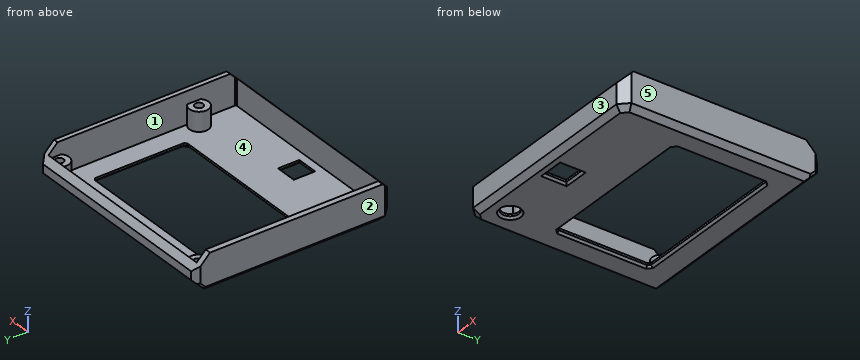
from build123d import *

# Parameters (mm, degrees)
PAD_DEPTH       = 17
POCKET_DEPTH    = 15
SKETCH002_R     = 4
SKETCH002_W     = 74.5
SKETCH002_H     = 43.5
SKETCH002_W_2   = 10
SKETCH002_H_2   = 10
POCKET001_DEPTH = 482
SKETCH003_R     = 4.5
SKETCH003_R_2   = 1.95
SKETCH003_R_3   = 3.5
PAD001_DEPTH    = 9
POCKET002_DEPTH = 99
PAD002_DEPTH    = 99
CHAMFER_SIZE    = 2.5
CHAMFER001_SIZE = 1


with BuildPart() as part:
    # Sketch → Pad (new body)
    with BuildSketch(Plane.XY):
        Polygon((0, 0), (99, 0), (99, -89), (95, -93), (4, -93), (0, -89), align=None)
    extrude(amount=PAD_DEPTH)

    # Sketch001 → Pocket (cut)
    with BuildSketch(Plane.XY.offset(17)):
        Polygon((2.75, -2.75), (96.75, -2.75), (96.75, -90.25), (96.25, -90.75), (3.25, -90.75), (2.75, -90.25), align=None)
    extrude(amount=-POCKET_DEPTH, mode=Mode.SUBTRACT)

    # Sketch002 (on Sketch) → Pocket001 (cut)
    with BuildSketch(Plane.XY.offset(482)):
        with Locations((12.75, -82)):
            Circle(SKETCH002_R)
        with Locations((49.75, -38.25)):
            Rectangle(SKETCH002_W, SKETCH002_H)
        with Locations((46.5, -82)):
            Rectangle(SKETCH002_W_2, SKETCH002_H_2)
    extrude(amount=-POCKET001_DEPTH, mode=Mode.SUBTRACT)

    # Sketch003 → Pad001 (join)
    with BuildSketch(Plane.XY.offset(2)):
        with Locations((5.5, -5.5)):
            Circle(SKETCH003_R)
        with Locations((5.5, -5.5)):
            Circle(SKETCH003_R_2, mode=Mode.SUBTRACT)
        with Locations((93.5, -5.5)):
            Circle(SKETCH003_R)
        with Locations((93.5, -5.5)):
            Circle(SKETCH003_R_2, mode=Mode.SUBTRACT)
        with Locations((5.5, -71)):
            Circle(SKETCH003_R_3)
        with Locations((5.5, -71)):
            Circle(SKETCH003_R_2, mode=Mode.SUBTRACT)
        with Locations((93.5, -71)):
            Circle(SKETCH003_R)
        with Locations((93.5, -71)):
            Circle(SKETCH003_R_2, mode=Mode.SUBTRACT)
    extrude(amount=PAD001_DEPTH)

    # Sketch004 → Pocket002 (cut)
    with BuildSketch(Plane.YZ):
        Polygon((-93, 24.5), (-93, 12), (-80.5, 24.5), align=None)
        Polygon((-12.5, 22.5), (0, 10), (0, 22.5), align=None)
        Polygon((0, 0), (0, 6), (-6, 0), align=None)
    extrude(amount=POCKET002_DEPTH, mode=Mode.SUBTRACT)

    # Sketch005 → Pad002 (join)
    with BuildSketch(Plane.YZ):
        Polygon((0, 6), (-6, 0), (-9.54, 0), (0, 9.54), align=None)
    extrude(amount=PAD002_DEPTH)

    # Chamfer
    chamfer_edges = [part.edges().sort_by_distance(p)[0] for p in [
        (99, -47.5, 0),
        (97, -91, 0),
        (49.5, -93, 0),
        (2, -91, 0),
        (0, -47.5, 0),
        (99, 0, 8),
        (0, 0, 8),
    ]]
    chamfer(chamfer_edges, length=CHAMFER_SIZE)

    # Chamfer001
    chamfer001_edges = [part.edges().sort_by_distance(p)[0] for p in [
        (99, -3, 3),
        (0, -3, 3),
        (12.5, -38.25, 0),
        (49.75, -16.5, 0),
        (49.75, -60, 0),
        (87, -38.25, 0),
        (51.5, -82, 0),
        (46.5, -87, 0),
        (41.5, -82, 0),
        (46.5, -77, 0),
        (8.75, -82, 0),
        (12.5, -60, 1),
        (87, -16.5, 1),
        (12.5, -16.5, 1),
        (87, -60, 1),
    ]]
    chamfer(chamfer001_edges, length=CHAMFER001_SIZE)


solid = part.part
Build history of the part. All positions in model axes, mm. Face numbers are marked on the shaded views. A direction names the side the tool comes from. Coordinates: 2 decimals unless noted, no trailing zeros. Order: outer loops, then holes, each group sorted by start corner. A loop starts at its lowest first (then second) coordinate and runs counter-clockwise, first axis right, second up. Notation, with made-up numbers: (76.5, 68) - (122.5, 68) arc R23 ccw to (122.5, 91) - close; hole circle Ø2 at (16, 21). An arc over 180 degrees is marked (long way). Write item = value, one per line. Start each with the question number.
1) Two-plate mould, pull along Y, no slides. Class the marked faces 3, 4 and 5: pulls with the +Y half, pulls with the -Y half, needs draft (parallel to the pull), parting line crosses it, or undercut.
2) 3-axis set-ups, long thin cutter, end or side, ignore diameter. For the marked faces 1 and 2: which of +Z, -Z, +X, -X, +Y, -Y reach the whole face in a straight line?
3) Saw through at D-D on z = 8.75. Write the cut outline in (x, y).
4) Saw through at A-A on x = 25.5. Write the cut outline in (y, z).
5) Wall check: line 1 along X through (y, z) = (-57, 11.5); line 2 along Y through (x, z) = (93.5, 4.25). Give the ranges that are in metal, low to high. Write a range as from..to.
6) Flat gauge pins, fed straight in: pin 1 Ø12 at (x, y) = (79, -72.5) entering from +Z; pin 2 Ø0.8 at (x, z) = (48.5, 1.5) entering from -Y; pin 3 Ø0.5 at (y, z) = (-30, 1.5) entering from +X. Where does each tip first touch, or does it go through?
7) Saw through at B-B on y = -56. Write the cut outline in (x, z).
8) Saw through at C-C on y = -82. Write the cut outline in (x, z), then the cut area to 3 significant figures.
From the geometry:
q1.face_3 = pulls with the -Y half
q1.face_4 = undercut
q1.face_5 = needs draft
q2.face_1 = +Z
q2.face_2 = +Z, -Z, -X, +Y, -Y
q3.outline = (0, -89) - (4, -93) - (95, -93) - (99, -89) - (99, -2.5) - (96.5, 0) - (2.5, 0) - (0, -2.5) - close; hole (2.75, -90.25) - (3.25, -90.75) - (96.25, -90.75) - (96.75, -90.25) - (96.75, -74.11) arc R4.5 cw (long way) to (96.75, -67.89) - (96.75, -8.61) arc R4.5 cw to (89.94, -2.75) - (9.06, -2.75) arc R4.5 cw to (2.75, -9.06) - (2.75, -68.83) arc R3.5 cw (long way) to (2.75, -73.17) - close; hole circle Ø3.9 at (5.5, -71); hole circle Ø3.9 at (5.5, -5.5); hole circle Ø3.9 at (93.5, -71); hole circle Ø3.9 at (93.5, -5.5)
q4.outline = (-93, 2.5) - (-90.5, 0) - (-61, 0) - (-60, 1) - (-60, 2) - (-90.75, 2) - (-90.75, 14.25) - (-93, 12) - close; (-16.5, 1) - (-15.5, 0) - (-6, 0) - (0, 6) - (0, 10) - (-2.75, 12.75) - (-2.75, 6.79) - (-7.54, 2) - (-16.5, 2) - close
q5.line_1 = 0..2.75, 96.75..99
q5.line_2 = -93..-90.75, -75.5..-72.95, -69.05..-66.5, -10..-7.45, -5.29..-1.75
q6.pin_1 = 2
q6.pin_2 = -92.4
q6.pin_3 = 98.25
q7.outline = (0, 2.5) - (2.5, 0) - (11.5, 0) - (12.5, 1) - (12.5, 2) - (2.75, 2) - (2.75, 17) - (0, 17) - close; (87, 1) - (88, 0) - (96.5, 0) - (99, 2.5) - (99, 17) - (96.75, 17) - (96.75, 2) - (87, 2) - close
q8.outline = (0, 2.5) - (2.5, 0) - (7.75, 0) - (8.75, 1) - (8.75, 2) - (2.75, 2) - (2.75, 17) - (0, 17) - close; (16.75, 1) - (17.75, 0) - (40.5, 0) - (41.5, 1) - (41.5, 2) - (16.75, 2) - close; (51.5, 1) - (52.5, 0) - (96.5, 0) - (99, 2.5) - (99, 17) - (96.75, 17) - (96.75, 2) - (51.5, 2) - close
q8.area = 229 mm^2
